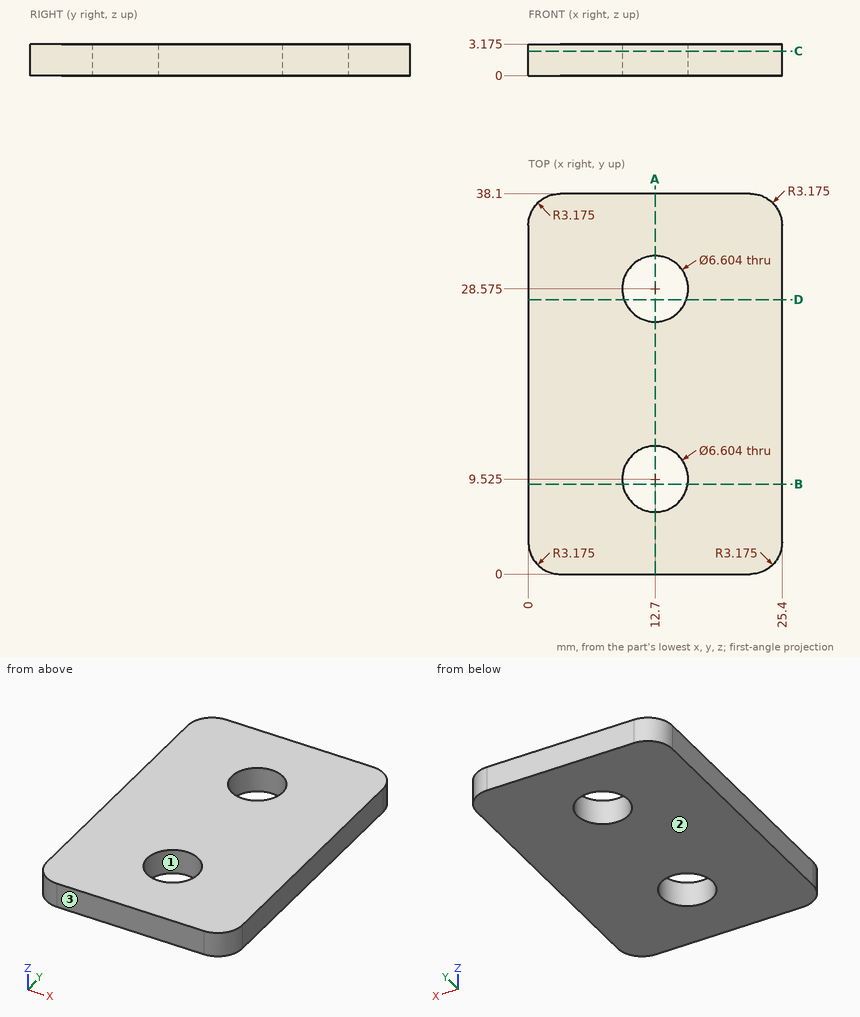
Here's the drawing with two shaded views (mm, measured from the low corner). I have some questions. Give positions to 0.01 mm unless a question says otherwise; leave off trailing zeros. Write each loop counter-clockwise with the first axis right and the second up, starting at its lowest first coordinate (ties: lowest second). Pieces come first, ordered by that corner, then holes. Notation, with made-up numbers: (32.25, 72.5) -> (54.25, 72.5) arc R26 cw to (54.25, 98.5) -> close; hole circle Ø11 at (58.5, 30.5). An arc over 180 degrees is marked (long way). Answer as a JSON object with one key per item and string values. Group by question number.
Item 1: We'd pull the mould along Y, two halves only. Please class the marked faces 1, 2 and 3: +Y half, -Y half, draft (parallel to the pull), parting line (faces both ways), or undercut.
Item 2: Suppose I cut it at C-C (z = 2.45). Please give me the cut outline in (x, y) (3 decimals).
Item 3: Suppose I cut it at A-A (x = 12.7). Please give me the cut outline in (y, z) (3 decimals).
Item 4: I'm going to push a flat-ended pin straight in: P1, Ø4, axis at x = 12.7, y = 9.525, coming from the +Z side. Where does the tip first touch, or does it pass through?
Item 5: Please list where these lines run through material, in increasing order: line 1 (Y direction, x = 12.7, z = 1.65); line 2 (Y direction, x = 12, z = 2.7); line 3 (X direction, y = 26, z = 1). Write a range as [from, to].
Item 6: Suppose I cut it at B-B (y = 9). Please give me the cut outline in (x, z) (3 decimals).
Item 7: Suppose I cut it at D-D (y = 27.5). Please give me the cut outline in (x, z) (3 decimals).
Findings:
{
 "1": {"face 1": "undercut", "face 2": "draft", "face 3": "-Y half"},
 "2": {"outline": "(0, 3.175) arc R3.175 ccw to (3.175, 0) -> (22.225, 0) arc R3.175 ccw to (25.4, 3.175) -> (25.4, 34.925) arc R3.175 ccw to (22.225, 38.1) -> (3.175, 38.1) arc R3.175 ccw to (0, 34.925) -> close; hole circle Ø6.604 at (12.7, 9.525); hole circle Ø6.604 at (12.7, 28.575)"},
 "3": {"outline": "(0, 0) -> (6.223, 0) -> (6.223, 3.175) -> (0, 3.175) -> close; (12.827, 0) -> (25.273, 0) -> (25.273, 3.175) -> (12.827, 3.175) -> close; (31.877, 0) -> (38.1, 0) -> (38.1, 3.175) -> (31.877, 3.175) -> close"},
 "4": {"P1": "passes through"},
 "5": {"line 1": "y = [0, 6.22], [12.83, 25.27], [31.88, 38.1]", "line 2": "y = [0, 6.3], [12.75, 25.35], [31.8, 38.1]", "line 3": "x = [0, 10.63], [14.77, 25.4]"},
 "6": {"outline": "(0, 0) -> (9.44, 0) -> (9.44, 3.175) -> (0, 3.175) -> close; (15.96, 0) -> (25.4, 0) -> (25.4, 3.175) -> (15.96, 3.175) -> close"},
 "7": {"outline": "(0, 0) -> (9.578, 0) -> (9.578, 3.175) -> (0, 3.175) -> close; (15.822, 0) -> (25.4, 0) -> (25.4, 3.175) -> (15.822, 3.175) -> close"}
}
